The model under review builds one solid part; all positions refer to its coordinate system, in mm. A direction names the side the tool comes from. Give positions to 0.01 mm unless a question says otherwise; leave off trailing zeros. Loops run counter-clockwise (first coordinate to the right, second up) from the corner with the lowest first, then second, coordinate; pieces in that order, holes last. Notation, with made-up numbers: M 57,-23.75 L 73,-23.75 A26 ccw 73,-8.75 Z; hole C -11.75,45.5 d1. An arc over 180 degrees is marked long. Put each result on its own line as item: value. Start each with the question number.
```python
from build123d import *

# Parameters (mm, degrees)
F0_R     = 10
F1_DEPTH = 76.230982
F2_W     = 41.696184
F2_H     = 43.047138
F2_R     = 10
F3_DEPTH = 25


with BuildPart() as f1:
    # F0 (on Top) → F1 (new body)
    with BuildSketch(Plane.XY):
        Circle(F0_R)
    extrude(amount=F1_DEPTH)

    # F2 (on face) → F3 (join)
    with BuildSketch(Plane.XY):
        Rectangle(F2_W, F2_H)
        Circle(F2_R, mode=Mode.SUBTRACT)
    extrude(amount=F3_DEPTH)


solid = f1.part
```
Item 1: Clearance check with flat-ended pins moving along their axes: pin 1 Ø10 at (x, z) = (2, 35.5) entering from -Y; pin 2 Ø4 at (y, z) = (3.5, 43) entering from -X; pin 3 Ø8 at (x, y) = (13, -15.5) entering from +Z. State where each tip first meets the part, or that it passes through.
Item 2: Consider section A-A, the plane x = 0. Write out the cut boundary in (y, z), plus the area to 3 significant figures.
Item 3: To check wall thickness, follow L1, parallel to Z at x = -15, y = 2.5; L2, parallel to X at y = -9, z = 59.5; L3, parallel to X at y = -0.5, z = 67.5. State the ranges of each line that lie inside material, in increasing order. Write a range as [from, to].
Item 4: Consider section C-C, the plane z = 58. Write out the cut boundary in (x, y), plus the area to 3 significant figures.
Item 5: Tool access review of faces 1 (the flat face through (9, 5, 25)), 2 (the flat face through (-20.848, 0, 12)): name each direction out of +Z, -Z, +X, -X, +Y, -Y from which nothing blocks a thin tool from reaching the whole face with its end or side.
Item 6: Consider section B-B, the plane y = 0. Write out the cut boundary in (x, z).
Item 7: Consider section D-D, the plane x = -17.5. Write out the cut boundary in (y, z), plus the area to 3 significant figures.
Report:
1. pin 1: y = -10
1. pin 2: x = -9.89
1. pin 3: z = 25
2. outline: M -21.52,0 L 21.52,0 L 21.52,25 L 10,25 L 10,76.23 L -10,76.23 L -10,25 L -21.52,25 Z
2. area: 2,100 mm²
3. L1: [0, 25]
3. L2: [-4.36, 4.36]
3. L3: [-9.99, 9.99]
4. outline: C 0,0 d20
4. area: 314 mm²
5. face 1: +Z
5. face 2: +Z, -Z, -X, +Y, -Y
6. outline: M -20.85,0 L 20.85,0 L 20.85,25 L 10,25 L 10,76.23 L -10,76.23 L -10,25 L -20.85,25 Z
7. outline: M -21.52,0 L 21.52,0 L 21.52,25 L -21.52,25 Z
7. area: 1,080 mm²
